from build123d import *

# Parameters (mm, degrees)
SKETCH_1_W             = 23.5
SKETCH_1_H             = 12
EXTRUDE_1_DEPTH        = 175
HOLE_WIZARD_M6_1_D     = 5
HOLE_WIZARD_M6_1_DEPTH = 15
HOLE_WIZARD_M6_1_TIP   = 1.502151548
HOLE_WIZARD_M6_2_D     = 5
HOLE_WIZARD_M6_2_DEPTH = 15
HOLE_WIZARD_M6_2_TIP   = 1.502151548
HOLE_WIZARD_M4_1_D     = 3.3
HOLE_WIZARD_M4_1_DEPTH = 10.1
HOLE_WIZARD_M4_1_TIP   = 0.991420021
HOLE_WIZARD_M6_3_D     = 5
HOLE_WIZARD_M6_3_DEPTH = 15
HOLE_WIZARD_M6_3_TIP   = 1.502151548


with BuildPart() as part:
    # 草图1 → 凸台-拉伸1 (new, symmetric)
    with BuildSketch(Plane(origin=(0, 0, 0), x_dir=(0, 0, -1), z_dir=(1, 0, 0))):
        with BuildLine():
            Line((-14, 15), (-11.5, 15))
            Line((-11.5, 15), (-11.5, 13.5))
            Line((-11.5, 13.5), (-11.4, 13.5))
            ThreePointArc((-11.4, 13.5), (-11.117157288, 13.382842712), (-11, 13.1))
            Line((-11, 13.1), (-11, 12))
            Line((-11, 12), (-9.5, 12))
            Line((-9.5, 12), (-9.5, 15))
            Line((-9.5, 15), (-8, 15))
            Line((-8, 15), (-8, 12.5))
            Line((-8, 12.5), (-5, 12.5))
            Line((-5, 12.5), (-5, 15))
            Line((-5, 15), (5, 15))
            Line((5, 15), (5, 12.5))
            Line((5, 12.5), (8, 12.5))
            Line((8, 12.5), (8, 15))
            Line((8, 15), (9.5, 15))
            Line((9.5, 15), (9.5, 12))
            Line((9.5, 12), (11, 12))
            Line((11, 12), (11, 13.1))
            ThreePointArc((11, 13.1), (11.117157288, 13.382842712), (11.4, 13.5))
            Line((11.4, 13.5), (11.5, 13.5))
            Line((11.5, 13.5), (11.5, 15))
            Line((11.5, 15), (14, 15))
            ThreePointArc((14, 15), (14.707106781, 14.707106781), (15, 14))
            Line((15, 14), (15, 8))
            Line((15, 8), (12.5, 8))
            Line((12.5, 8), (12.5, 5))
            Line((12.5, 5), (15, 5))
            Line((15, 5), (15, -5))
            Line((15, -5), (12.5, -5))
            Line((12.5, -5), (12.5, -8))
            Line((12.5, -8), (15, -8))
            Line((15, -8), (15, -14))
            ThreePointArc((15, -14), (14.707106781, -14.707106781), (14, -15))
            Line((14, -15), (11.5, -15))
            Line((11.5, -15), (11.5, -13.5))
            Line((11.5, -13.5), (11.4, -13.5))
            ThreePointArc((11.4, -13.5), (11.117157288, -13.382842712), (11, -13.1))
            Line((11, -13.1), (11, -12))
            Line((11, -12), (9.5, -12))
            Line((9.5, -12), (9.5, -15))
            Line((9.5, -15), (8, -15))
            Line((8, -15), (8, -12.5))
            Line((8, -12.5), (5, -12.5))
            Line((5, -12.5), (5, -15))
            Line((5, -15), (-5, -15))
            Line((-5, -15), (-5, -12.5))
            Line((-5, -12.5), (-8, -12.5))
            Line((-8, -12.5), (-8, -15))
            Line((-8, -15), (-9.5, -15))
            Line((-9.5, -15), (-9.5, -12))
            Line((-9.5, -12), (-11, -12))
            Line((-11, -12), (-11, -13.1))
            ThreePointArc((-11, -13.1), (-11.117157288, -13.382842712), (-11.4, -13.5))
            Line((-11.4, -13.5), (-11.5, -13.5))
            Line((-11.5, -13.5), (-11.5, -15))
            Line((-11.5, -15), (-14, -15))
            ThreePointArc((-14, -15), (-14.707106781, -14.707106781), (-15, -14))
            Line((-15, -14), (-15, 14))
            ThreePointArc((-15, 14), (-14.707106781, 14.707106781), (-14, 15))
        make_face()
        with BuildLine():
            Line((12, -10.5), (12, -8.5))
            ThreePointArc((12, -8.5), (11.853553391, -8.146446609), (11.5, -8))
            Line((11.5, -8), (-11.5, -8))
            ThreePointArc((-11.5, -8), (-11.853553391, -8.146446609), (-12, -8.5))
            Line((-12, -8.5), (-12, -10.5))
            ThreePointArc((-12, -10.5), (-11.853553391, -10.853553391), (-11.5, -11))
            Line((-11.5, -11), (11.5, -11))
            ThreePointArc((11.5, -11), (11.853553391, -10.853553391), (12, -10.5))
        make_face(mode=Mode.SUBTRACT)
        with BuildLine():
            Line((-11.5, 11), (11.5, 11))
            ThreePointArc((11.5, 11), (11.853553391, 10.853553391), (12, 10.5))
            Line((12, 10.5), (12, 8.5))
            ThreePointArc((12, 8.5), (11.853553391, 8.146446609), (11.5, 8))
            Line((11.5, 8), (-11.5, 8))
            ThreePointArc((-11.5, 8), (-11.853553391, 8.146446609), (-12, 8.5))
            Line((-12, 8.5), (-12, 10.5))
            ThreePointArc((-12, 10.5), (-11.853553391, 10.853553391), (-11.5, 11))
        make_face(mode=Mode.SUBTRACT)
        Rectangle(SKETCH_1_W, SKETCH_1_H, mode=Mode.SUBTRACT)
    extrude(amount=EXTRUDE_1_DEPTH, both=True)

    # M6 螺纹孔1
    with Locations(Plane.XZ.offset(15)):
        with Locations((-155, 0), (-140, 0), (155, 0), (140, 0)):
            Hole(HOLE_WIZARD_M6_1_D / 2, depth=HOLE_WIZARD_M6_1_DEPTH)
            with Locations((0, 0, -(HOLE_WIZARD_M6_1_DEPTH + HOLE_WIZARD_M6_1_TIP / 2))):  # 118° drill point
                Cone(0, HOLE_WIZARD_M6_1_D / 2, HOLE_WIZARD_M6_1_TIP, mode=Mode.SUBTRACT)

    # M6 螺纹孔2
    with Locations(Plane(origin=(0, 15, 0), x_dir=(-1, 0, 0), z_dir=(0, 1, 0))):
        with Locations((155, 0), (140, 0), (-155, 0), (-140, 0)):
            Hole(HOLE_WIZARD_M6_2_D / 2, depth=HOLE_WIZARD_M6_2_DEPTH)
            with Locations((0, 0, -(HOLE_WIZARD_M6_2_DEPTH + HOLE_WIZARD_M6_2_TIP / 2))):  # 118° drill point
                Cone(0, HOLE_WIZARD_M6_2_D / 2, HOLE_WIZARD_M6_2_TIP, mode=Mode.SUBTRACT)

    # M4 螺纹孔1
    with Locations(Plane(origin=(0, 15, 0), x_dir=(-1, 0, 0), z_dir=(0, 1, 0))):
        with Locations((100, 0), (0, 0), (-100, 0)):
            Hole(HOLE_WIZARD_M4_1_D / 2, depth=HOLE_WIZARD_M4_1_DEPTH)
            with Locations((0, 0, -(HOLE_WIZARD_M4_1_DEPTH + HOLE_WIZARD_M4_1_TIP / 2))):  # 118° drill point
                Cone(0, HOLE_WIZARD_M4_1_D / 2, HOLE_WIZARD_M4_1_TIP, mode=Mode.SUBTRACT)

    # M6 螺纹孔3
    with Locations(Plane.XZ.offset(15)):
        with Locations((-105, 0), (105, 0)):
            Hole(HOLE_WIZARD_M6_3_D / 2, depth=HOLE_WIZARD_M6_3_DEPTH)
            with Locations((0, 0, -(HOLE_WIZARD_M6_3_DEPTH + HOLE_WIZARD_M6_3_TIP / 2))):  # 118° drill point
                Cone(0, HOLE_WIZARD_M6_3_D / 2, HOLE_WIZARD_M6_3_TIP, mode=Mode.SUBTRACT)


solid = part.part
Geometry: final body of the model. Coordinates: model frame, mm. A direction names the side the tool comes from. Coordinates: 2 decimals unless noted, no trailing zeros. Order: outer loops, then holes, each group sorted by start corner. A loop starts at its lowest first (then second) coordinate and runs counter-clockwise, first axis right, second up. Notation, with made-up numbers: M 32.25,35.25 L 85.25,35.25 A7 ccw 85.25,46.25 Z; hole C 70.5,-21.5 d9. An arc over 180 degrees is marked long. One line per question, with ' | ' between items. Start each with the question number.
Item 1: Cut plane B-B, the plane x = 69. Count the separate pieces of the cut face and the enclosed holes in it, then the cut area to 3 significant figures.
Item 2: Draft query along Y for faces 3 (the flat face through (2, -15, 0)), 4 (the flat face through (2, 8, 0)), 5 (the flat face through (2, 11, 0)), 6 (the flat face through (-175, 7, 0)). Return one class per face: released by +Y, released by -Y, zero draft, split by the parting line, or undercut.
Item 3: Pin query (flat end, axial travel): pin 1 Ø3 at (x, z) = (100, 0) entering from +Y; pin 2 Ø0.9 at (x, y) = (80, 7) entering from -Z; pin 3 Ø3 at (x, z) = (140, 0) entering from +Y. Return the tip coordinate at first contact, or that it passes through.
Item 4: Ray query, probe 1 along Y at (x, z) = (-88.5, -9.75); probe 2 along Z at (x, y) = (155, 14.05); probe 3 along Y at (x, z) = (-21.5, -4). Return the intervals inside material, ascending. Write a range as [from, to].
Item 5: Set-up query: faces 1 (the flat face through (2, -11, 0)), 2 (the flat face through (2, -11, -15)). Return all of +Z, -Z, +X, -X, +Y, -Y with unobstructed straight access to the full face (end or side cutting, diameter ignored); none if empty.
Item 6: Cut plane A-A, the plane y = 0.5. Return the cut outline in (x, z), then the cut area to 4 significant figures.
A:
1) separate pieces: 1 | enclosed holes: 3 | area: 407 mm2
2) face 3: released by -Y | face 4: undercut | face 5: undercut | face 6: zero draft
3) pin 1: stops at y = -6 | pin 2: stops at z = -12.5 | pin 3: passes through
4) probe 1: y = [-12, -11], [-8, -6], [6, 8], [11, 12] | probe 2: z = [-15, -11.5], [-9.5, -8], [-5, -2.5], [2.5, 5], [8, 9.5], [11.5, 15] | probe 3: y = [-15, -11], [-8, -6], [6, 8], [11, 15]
5) face 1: +X, -X | face 2: -Z, +X, -X, +Y, -Y
6) outline: M -175,-15 L 175,-15 L 175,-11.75 L -175,-11.75 Z; M -175,11.75 L 175,11.75 L 175,15 L -175,15 Z | area: 2,275 mm2
